Design review of the part shown in the three views and the two pictorial views. Dimensions are in mm from the part's minimum x, y and z. Give positions to 0.01 mm unless a question says otherwise; leave off trailing zeros. Loops run counter-clockwise (first coordinate to the right, second up) from the corner with the lowest first, then second, coordinate; pieces in that order, holes last. Notation, with made-up numbers: (-25, -21) -> (15, -21) arc R17 cw to (15, 8) -> close; hole circle Ø2 at (49.25, 58). An arc over 180 degrees is marked (long way). Answer as CSV lines item,"result".
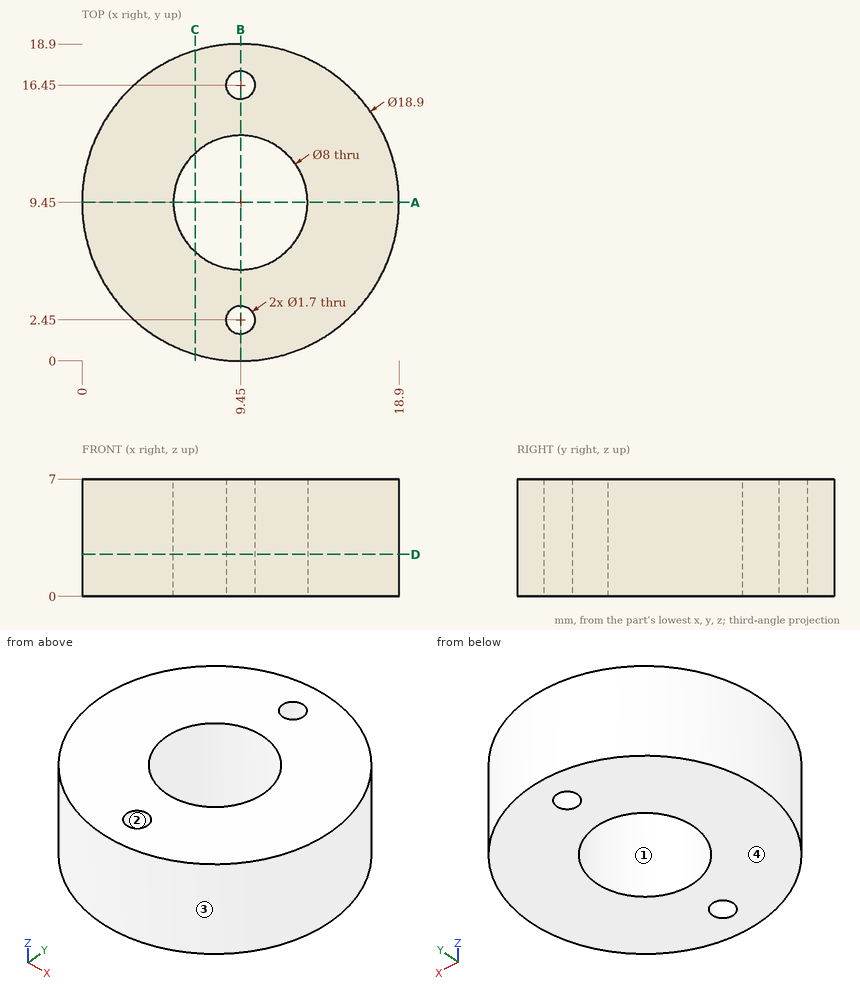
Q1. We need section B-B, the plane x = 9.45. State the section outline as (y, z) points, and give its area (3 significant figures).
Filled sheet:
outline,"(0, 0) -> (1.6, 0) -> (1.6, 7) -> (0, 7) -> close; (3.3, 0) -> (5.45, 0) -> (5.45, 7) -> (3.3, 7) -> close; (13.45, 0) -> (15.6, 0) -> (15.6, 7) -> (13.45, 7) -> close; (17.3, 0) -> (18.9, 0) -> (18.9, 7) -> (17.3, 7) -> close"
area,"52.5 mm^2"
Q2. We need section C-C, the plane x = 6.75. State the section outline as (y, z) points.
Filled sheet:
outline,"(0.39, 0) -> (6.5, 0) -> (6.5, 7) -> (0.39, 7) -> close; (12.4, 0) -> (18.51, 0) -> (18.51, 7) -> (12.4, 7) -> close"
Q3. The part is to be moulded in two halves that separate along X. For the marked faces 1, 2, 3 and 4, say which applies: pulls with the +X half, pulls with the -X half, needs draft (parallel to the pull), parting line crosses it, or undercut.
Filled sheet:
face 1,"undercut"
face 2,"undercut"
face 3,"parting line crosses it"
face 4,"needs draft"
Q4. Clearance check with flat-ended pins moving along their axes: pin 1 Ø3 at (y, z) = (16.5, 6) entering from -X; pin 2 Ø1 at (x, z) = (4.5, 1.5) entering from +Y; pin 3 Ø3 at (x, z) = (16.5, 3.5) entering from +Y. State where each tip first meets the part, or that it passes through.
Filled sheet:
pin 1,"stops at x = 1.8"
pin 2,"stops at y = 17.79"
pin 3,"stops at y = 17.1"
Q5. To check wall thickness, follow probe 1 along Y at (x, z) = (9.45, 4.25); probe 2 along Y at (x, z) = (7.25, 0.75); probe 3 along X at (y, z) = (6.5, 0.5). State the ranges of each line that lie inside material, in increasing order. Write a range as from..to.
Filled sheet:
probe 1,"y = 0..1.6, 3.3..5.45, 13.45..15.6, 17.3..18.9"
probe 2,"y = 0.26..6.11, 12.79..18.64"
probe 3,"x = 0.47..6.75, 12.15..18.43"
Q6. We need section A-A, the plane y = 9.45. State the section outline as (x, z) points.
Filled sheet:
outline,"(0, 0) -> (5.45, 0) -> (5.45, 7) -> (0, 7) -> close; (13.45, 0) -> (18.9, 0) -> (18.9, 7) -> (13.45, 7) -> close"
Q7. We need section D-D, the plane z = 2.5. State the section outline as (x, y) points.
Filled sheet:
outline,"circle Ø18.9 at (9.45, 9.45); hole circle Ø8 at (9.45, 9.45); hole circle Ø1.7 at (9.45, 2.45); hole circle Ø1.7 at (9.45, 16.45)"
